Design review of the part built by this model. Coordinates are the model's own, in mm. Coordinates: 2 decimals unless noted, no trailing zeros. Write each loop counter-clockwise with the first axis right and the second up, starting at its lowest first coordinate (ties: lowest second). Pieces come first, ordered by that corner, then holes. Notation, with made-up numbers: (44, 24) - (94, 24) arc R18 ccw to (94, 35) - close; hole circle Ø7 at (31, 72). An arc over 180 degrees is marked (long way). One line per item, written item: value.
from build123d import *

# Parameters (mm, degrees)
SKETCH2_R          = 1
CUT_EXTRUDE1_DEPTH = 5


with BuildPart() as part:
    # Sketch1 → Revolve1 (revolve)
    with BuildSketch(Plane(origin=(0, 0, 0), x_dir=(0, 0, -1), z_dir=(1, 0, 0))):
        with BuildLine():
            Line((-7, -19.250050998), (0, -19.250050998))
            Line((0, -19.250050998), (0, 20.749949002))
            Line((0, 20.749949002), (-12.5, 20.749949002))
            ThreePointArc((-12.5, 20.749949002), (-14.267766953, 20.017715955), (-15, 18.249949002))
            Line((-15, 18.249949002), (-15, 15.749949002))
            ThreePointArc((-15, 15.749949002), (-9.025461564, -1.298727927), (-7, -19.250050998))
        make_face()
    revolve(axis=Axis((0, 28.85, 0), (0, -1, 0)))

    # Sketch2 → Cut-Extrude1 (cut)
    with BuildSketch(Plane.XZ.offset(19.250050998)):
        with Locations(Location((0, 0, 0), (0, 0, 270))):
            Circle(SKETCH2_R)
    extrude(amount=-CUT_EXTRUDE1_DEPTH, mode=Mode.SUBTRACT)


solid = part.part
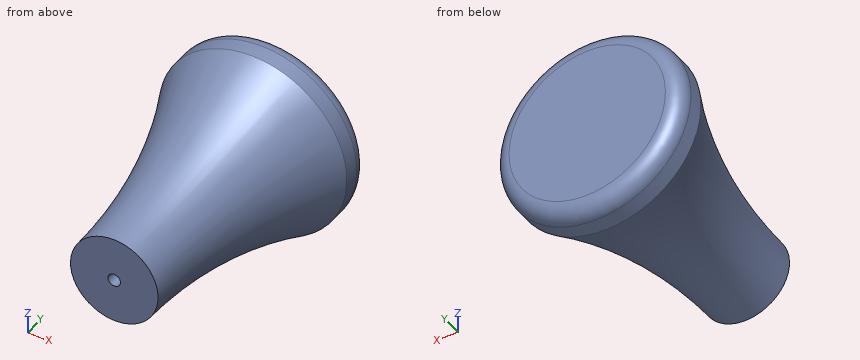
1. Consider section D-D, the plane y = 11. Write out the cut boundary in (x, z).
Answer block:
outline: circle Ø25.79 at (0, 0)
2. Consider section A-A, the plane z = 0. Write out the cut boundary in (x, y) (1 decimal).
Answer block:
outline: (-15, 15.7) arc R80.6 cw to (-7, -19.3) - (-1, -19.3) - (-1, -14.3) - (1, -14.3) - (1, -19.3) - (7, -19.3) arc R80.6 cw to (15, 15.7) - (15, 18.2) arc R2.5 ccw to (12.5, 20.7) - (-12.5, 20.7) arc R2.5 ccw to (-15, 18.2) - close
3. Wall thickness on line 1 along X through (y, z) = (-17.95, 0); line 2 along X through (y, z) = (-16.35, 0); line 3 along Z through (x, y) = (-8.5, 7): over which ranges is each line inside the solid? List them lowest first.
Answer block:
line 1: x = -7.01 to -1, 1 to 7.01
line 2: x = -7.05 to -1, 1 to 7.05
line 3: z = -7.59 to 7.59
4. Insertion check: pin 1 Ø12 at (x, z) = (-7.5, 10.5) entering from -Y; pin 2 Ø5 at (x, y) = (6, 15.5) entering from +Z; pin 3 Ø6 at (x, y) = (-4, -7) entering from +Z; pin 4 Ø1.5 at (x, y) = (5, 0.5) entering from +Z. Each pin has a flat end and moves straight along its axis. Give the tip position at first contact, or say it passes through.
Answer block:
pin 1: stops at y = -19.25
pin 2: stops at z = 14.58
pin 3: stops at z = 8.08
pin 4: stops at z = 8.51
5. Consider section B-B, the plane x = 0. Write out the cut boundary in (y, z) (1 decimal).
Answer block:
outline: (-19.3, -7) arc R80.6 cw to (15.7, -15) - (18.2, -15) arc R2.5 ccw to (20.7, -12.5) - (20.7, 12.5) arc R2.5 ccw to (18.2, 15) - (15.7, 15) arc R80.6 cw to (-19.3, 7) - (-19.3, 1) - (-14.3, 1) - (-14.3, -1) - (-19.3, -1) - close
6. Consider section C-C, the plane y = -17. Write out the cut boundary in (x, z), then the cut area to 3 significant figures.
Answer block:
outline: circle Ø14.06 at (0, 0); hole circle Ø2 at (0, 0)
area: 152 mm^2
